Part model, mm, in its own coordinate system. Face numbers are marked on the shaded views. A direction names the side the tool comes from. Round coordinates to 2 decimals unless told otherwise and drop trailing zeros. Write each loop counter-clockwise with the first axis right and the second up, starting at its lowest first coordinate (ties: lowest second). Pieces come first, ordered by that corner, then holes.
1) Saw through at C-C on z = -6.5. Write the cut outline in (x, y) (3 decimals).
2) Pull direction X, two halves, no side cores. Call the marked faces 3, 4 and 5: +X half, -X half, draft (parallel to the pull), parting line (faces both ways), or undercut.
3) Saw through at B-B on y = 37. Write the cut outline in (x, z).
4) Drill centre lines: L1, parallel to X at y = 30.5, z = -27; L2, parallel to Y at x = 59.5, z = -29 (3 decimals); L3, parallel to Z at x = -54, y = 24.5. Where is each one in solid material? Low to high.
5) Saw through at A-A on x = -11.5. Write the cut outline in (y, z) (3 decimals).
6) Flat gauge pins, fed straight in: pin 1 (2 mm diameter, centred on x = -48, z = -0.5, fed in from +Y) (3 decimals); pin 2 (2 mm diameter, centred on y = 6.1, z = 51.59, fed in from +X); pin 3 (3.5 mm diameter, centred on x = 65.913, y = 53.975, fed in from -Z); pin 4 (4.5 mm diameter, centred on x = 49.22, y = 60.89, fed in from +Z). Where does each tip first touch, or does it go through?
7) Which spindle directions (+Z, -Z, +X, -X, +Y, -Y) get a long thin tool onto all of the face, cutting with end or side? Do the marked faces 1 and 2. Say none if no direction does.
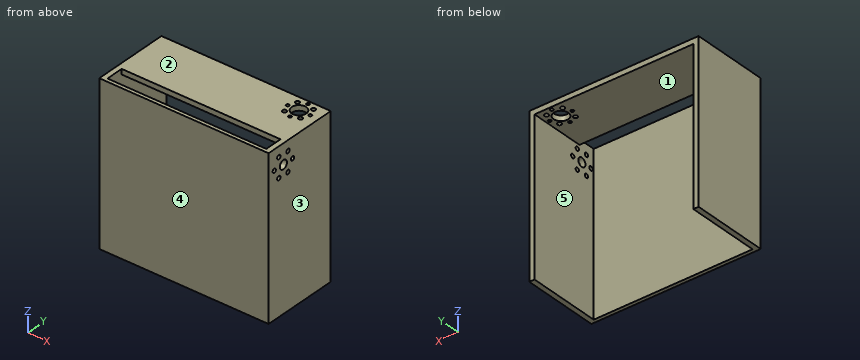
Autodesk Inventor part; units mm, degrees
ref_plane "YZ Plane" through (0, 0, 0) normal (1, 0, 0) x (0, 1, 0)
ref_plane "XZ Plane" through (0, 0, 0) normal (0, 1, 0) x (-1, 0, 0)
ref_plane "XY Plane" through (0, 0, 0) normal (0, 0, 1) x (1, 0, 0)
sketch "Sketch1" plane through (0, 0, 0) normal (0, 1, 0) x (-1, 0, 0)
  line L0 (73.3806, 68.834) -> (-73.3806, 68.834)
  line L1 (-73.3806, 68.834) -> (-73.3806, -68.834)
  line L2 (-73.3806, -68.834) -> (73.3806, -68.834)
  line L3 (73.3806, -68.834) -> (73.3806, 68.834)
  line L4 (73.3806, 68.834) -> (-73.3806, -68.834) construction
  line L5 (-73.3806, 68.834) -> (73.3806, -68.834) construction
  point P0 (0, 0)
  dimension "d0" = 146.7612
  dimension "d1" = 137.668
extrude "Extrusion1" add sketch "Sketch1" along normal blind 3.175
sketch "Sketch2" plane through (0, 3.175, 0) normal (0, 1, 0) x (1, 0, 0)
  line L0 (73.3806, 68.834) -> (-73.3806, 68.834)
  line L1 (-68.834, -68.834) -> (68.834, -68.834)
  line L2 (68.834, -68.834) -> (68.834, 68.834)
  line L3 (68.834, 68.834) -> (-68.834, 68.834)
  line L4 (-68.834, 68.834) -> (-68.834, -68.834)
  line L5 (-68.834, -68.834) -> (68.834, 68.834) construction
  line L6 (68.834, -68.834) -> (-68.834, 68.834) construction
  line L7 (73.3806, -68.834) -> (73.3806, 68.834)
  line L8 (73.3806, 68.834) -> (68.834, 68.834)
  line L9 (68.834, 68.834) -> (68.834, -68.834)
  line L10 (68.834, -68.834) -> (73.3806, -68.834)
  line L11 (73.3806, -68.834) -> (73.3806, 68.834)
  line L12 (-73.3806, 68.834) -> (-68.834, 68.834)
  line L13 (-68.834, 68.834) -> (-68.834, -68.834)
  line L14 (-68.834, -68.834) -> (-73.3806, -68.834)
  line L15 (-73.3806, -68.834) -> (-73.3806, 68.834)
  point P0 (0, 0)
  dimension "d4" = 137.668
extrude "Extrusion2" add sketch "Sketch2" along normal blind 63.5 contours L7 L10 L2 L0 | L4 L14 L15 L0
sketch "Sketch3" plane through (0, 3.175, 0) normal (0, 1, 0) x (1, 0, 0)
  line L0 (-68.834, -68.834) -> (68.834, -68.834)
  line L1 (68.834, 68.834) -> (68.834, -68.834)
  line L2 (-68.834, -68.834) -> (68.834, -68.834)
  line L3 (68.834, -68.834) -> (68.834, -64.2874)
  line L4 (68.834, -64.2874) -> (-68.834, -64.2874)
  line L5 (-68.834, -64.2874) -> (-68.834, -68.834)
  point P0 (0, 0)
  dimension "d7" = 4.5466
extrude "Extrusion3" add sketch "Sketch3" along normal blind 63.5
sketch "Sketch4" plane through (-73.3806, 0, 68.834) normal (0, 0, 1) x (1, 0, 0)
  line L0 (142.2146, 3.175) -> (4.5466, 3.175)
  line L1 (142.2146, 3.175) -> (142.2146, 66.675)
  line L2 (4.5466, 3.175) -> (142.2146, 3.175)
  line L3 (142.2146, 3.175) -> (142.2146, 18.415)
  line L4 (142.2146, 18.415) -> (4.5466, 18.415)
  line L5 (4.5466, 18.415) -> (4.5466, 3.175)
  point P0 (73.3806, 0)
  dimension "d10" = 15.24
extrude "Extrusion4" cut sketch "Sketch4" against normal blind 25.4
sketch "Sketch5" plane through (73.3806, 0, 68.834) normal (1, 0, 0) x (0, 0, -1)
  line L0 (4.5466, 66.675) -> (4.5466, 18.415)
  line L1 (4.5466, 20.7271) -> (4.5466, 3.175)
  line L2 (0, 3.175) -> (137.668, 3.175)
  line L3 (4.5466, 3.175) -> (29.9466, 3.175)
  line L4 (29.9466, 3.175) -> (29.9466, 28.575)
  line L5 (29.9466, 28.575) -> (4.5466, 28.575)
  line L6 (4.5466, 28.575) -> (4.5466, 3.175)
  circle A0 centre (17.2466, 15.875) radius 12.7
  circle A1 centre (17.2466, 15.875) radius 3.81
  line L7 (17.2466, 15.875) -> (17.2466, 25.654)
  circle A2 centre (17.2466, 25.654) radius 1.778
  circle A3 centre (8.7777, 20.7645) radius 1.778
  circle A4 centre (8.7777, 10.9855) radius 1.778
  circle A5 centre (17.2466, 6.096) radius 1.778
  circle A6 centre (25.7155, 10.9855) radius 1.778
  circle A7 centre (25.7155, 20.7645) radius 1.778
  point P0 (68.834, 0)
  dimension "d13" = 25.4
  dimension "d14" = 25.4
  dimension "d15" = 25.4
  dimension "d16" = 7.62
  dimension "d17" = 9.779
  dimension "d18" = 3.556
  dimension "d21" = 360
extrude "Extrusion5" cut sketch "Sketch5" against normal blind 25.4 contours A1 | A2 | A3 | A4 | A5 | A6 | A7
sketch "Sketch6" plane through (-73.3806, 0, 68.834) normal (0, 0, 1) x (1, 0, 0)
  line L0 (142.2146, 18.415) -> (142.2146, 66.675)
  line L1 (142.2146, 66.675) -> (116.8146, 66.675)
  line L2 (116.8146, 66.675) -> (116.8146, 41.275)
  line L3 (116.8146, 41.275) -> (142.2146, 41.275)
  line L4 (142.2146, 41.275) -> (142.2146, 66.675)
  circle A0 centre (129.5146, 53.975) radius 6.3627
  line L5 (129.5146, 53.975) -> (129.5146, 63.754)
  circle A1 centre (129.5146, 63.754) radius 1.3589
  circle A2 centre (119.7356, 53.975) radius 1.3589
  circle A3 centre (129.5146, 44.196) radius 1.3589
  circle A4 centre (139.2936, 53.975) radius 1.3589
  line L6 (129.5146, 53.975) -> (116.8146, 66.675)
  line L7 (129.5146, 53.975) -> (122.5998, 60.8898)
  circle A5 centre (122.5998, 60.8898) radius 1.778
  circle A6 centre (122.5998, 47.0602) radius 1.778
  circle A7 centre (136.4294, 47.0602) radius 1.778
  circle A8 centre (136.4294, 60.8898) radius 1.778
  point P0 (73.3806, 0)
  dimension "d25" = 25.4
  dimension "d26" = 25.4
  dimension "d27" = 12.7254
  dimension "d28" = 9.779
  dimension "d29" = 2.7178
  dimension "d32" = 360
  dimension "d34" = 9.779
  dimension "d35" = 3.556
  dimension "d38" = 360
extrude "Extrusion6" cut sketch "Sketch6" against normal blind 25.4 contours A1 | A0 L5 L6 | L6 L5 A0 | A5 L6 | L6 A5 | A2 | A3 | A4 | A6 | A7 | A8
properties part number "Box"
Completed:
1. outline: (-73.381, 0) - (73.381, 0) - (73.381, 66.675) - (68.834, 66.675) - (68.834, 3.175) - (-68.834, 3.175) - (-68.834, 66.675) - (-73.381, 66.675) - close
2. face 3: +X half
2. face 4: draft
2. face 5: undercut
3. outline: (-73.38, -68.83) - (-68.83, -68.83) - (-68.83, 64.29) - (68.83, 64.29) - (68.83, -68.83) - (73.38, -68.83) - (73.38, 68.83) - (-73.38, 68.83) - close
4. L1: x = -73.38 to -68.83, 68.83 to 73.38
4. L2: y = 0 to 3.175
4. L3: z = 64.29 to 68.83
5. outline: (0, -68.834) - (3.175, -68.834) - (3.175, 68.834) - (0, 68.834) - close; (18.415, 64.287) - (66.675, 64.287) - (66.675, 68.834) - (18.415, 68.834) - close
6. pin 1: stops at y = 3.175
6. pin 2: stops at x = -68.83
6. pin 3: stops at z = 64.29
6. pin 4: stops at z = 68.83
7. face 1: -Z, +Y
7. face 2: +Z, +X, -X, +Y, -Y
